from build123d import *

# Parameters (mm, degrees)
BOSS_EXTRUDE1_DEPTH = 11
SKETCH6_R           = 1
CUT_EXTRUDE7_DEPTH  = 11
SKETCH7_R           = 1
CUT_EXTRUDE8_DEPTH  = 11
SKETCH8_R           = 1
CUT_EXTRUDE9_DEPTH  = 10
CUT_EXTRUDE_START   = -6
CUT_EXTRUDE_1_DEPTH = 6
FILLET_1_R          = 2


with BuildPart() as part:
    # Sketch1 → Boss-Extrude1 (new body)
    with BuildSketch(Plane.XY):
        with BuildLine():
            Line((-54.397881045, 39.097965902), (-66.397881045, 39.097965902))
            Line((-66.397881045, 39.097965902), (-72.397881045, 33.097965902))
            Line((-72.397881045, 33.097965902), (-72.397881045, 25.597965902))
            Line((-72.397881045, 25.597965902), (-84.397881045, 25.597965902))
            ThreePointArc((-84.397881045, 25.597965902), (-85.104987826, 25.305072683), (-85.397881045, 24.597965902))
            Line((-85.397881045, 24.597965902), (-85.397881045, 18.597965902))
            ThreePointArc((-85.397881045, 18.597965902), (-85.104987826, 17.890859121), (-84.397881045, 17.597965902))
            Line((-84.397881045, 17.597965902), (-72.397881045, 17.597965902))
            Line((-72.397881045, 17.597965902), (-72.397881045, 10.097965902))
            Line((-72.397881045, 10.097965902), (-66.397881045, 4.097965902))
            Line((-66.397881045, 4.097965902), (-54.397881045, 4.097965902))
            ThreePointArc((-54.397881045, 4.097965902), (-53.690774263, 4.390859121), (-53.397881045, 5.097965902))
            Line((-53.397881045, 5.097965902), (-53.397881045, 9.097965902))
            ThreePointArc((-53.397881045, 9.097965902), (-53.690774263, 9.805072683), (-54.397881045, 10.097965902))
            Line((-54.397881045, 10.097965902), (-66.397881045, 10.097965902))
            Line((-66.397881045, 10.097965902), (-66.397881045, 33.097965902))
            Line((-66.397881045, 33.097965902), (-54.397881045, 33.097965902))
            ThreePointArc((-54.397881045, 33.097965902), (-53.690774263, 33.390859121), (-53.397881045, 34.097965902))
            Line((-53.397881045, 34.097965902), (-53.397881045, 38.097965902))
            ThreePointArc((-53.397881045, 38.097965902), (-53.690774263, 38.805072683), (-54.397881045, 39.097965902))
        make_face()
    extrude(amount=BOSS_EXTRUDE1_DEPTH)

    # Sketch6 → Cut-Extrude7 (cut)
    with BuildSketch(Plane(origin=(0, -0.303980624, 11), x_dir=(1, 0, 0), z_dir=(0, 0, 1))):
        with Locations((-59.897881045, 35.597965902)):
            Circle(SKETCH6_R)
    extrude(amount=-CUT_EXTRUDE7_DEPTH, mode=Mode.SUBTRACT)

    # Sketch7 → Cut-Extrude8 (cut)
    with BuildSketch(Plane(origin=(0, 0.204760049, 11), x_dir=(1, 0, 0), z_dir=(0, 0, 1))):
        with Locations((-59.897881045, 7.597965902)):
            Circle(SKETCH7_R)
    extrude(amount=-CUT_EXTRUDE8_DEPTH, mode=Mode.SUBTRACT)

    # Sketch8 → Cut-Extrude9 (cut)
    with BuildSketch(Plane(origin=(0, 25.597965902, 0), x_dir=(1, 0, 0), z_dir=(0, 1, 0))):
        with Locations(Location((-78.897881045, -2, 0), (0, 0, 270))):
            Circle(SKETCH8_R)
    extrude(amount=-CUT_EXTRUDE9_DEPTH, mode=Mode.SUBTRACT)

    # Эскиз1 → Вырез-Вытянуть1 (cut)
    with BuildSketch(Plane.XY.offset(11).offset(CUT_EXTRUDE_START)):
        with BuildLine():
            Line((-72.397881045, 17.597965902), (-72.397881045, 25.597965902))
            Line((-72.397881045, 25.597965902), (-84.397881045, 25.597965902))
            ThreePointArc((-84.397881045, 25.597965902), (-85.104987826, 25.305072683), (-85.397881045, 24.597965902))
            Line((-85.397881045, 24.597965902), (-85.397881045, 18.597965902))
            ThreePointArc((-85.397881045, 18.597965902), (-85.104987826, 17.890859121), (-84.397881045, 17.597965902))
            Line((-84.397881045, 17.597965902), (-72.397881045, 17.597965902))
        make_face()
    extrude(amount=CUT_EXTRUDE_1_DEPTH, mode=Mode.SUBTRACT)

    # Скругление1
    fillet_1_edges = [part.edges().sort_by_distance(p)[0] for p in [
        (-72.397881045, 10.097965902, 5.5),
        (-72.397881045, 33.097965902, 5.5),
        (-66.397881045, 39.097965902, 5.5),
        (-66.397881045, 4.097965902, 5.5),
    ]]
    fillet(fillet_1_edges, radius=FILLET_1_R)


solid = part.part
CAD build for the part. Positions are in the model's coordinates, mm. A direction names the side the tool comes from. Round coordinates to 2 decimals unless told otherwise and drop trailing zeros. Write each loop counter-clockwise with the first axis right and the second up, starting at its lowest first coordinate (ties: lowest second). Pieces come first, ordered by that corner, then holes. Notation, with made-up numbers: M 34.5,79.5 L 50.5,79.5 A17 cw 50.5,109.5 Z; hole C 56,60 d3. An arc over 180 degrees is marked long. Put each result on its own line as item: value. Start each with the question number.
1) Saw through at A-A, the plane z = 2. Count the separate pieces of the cut face and the enclosed holes in it, and give its area (3 significant figures).
2) Drill centre lines: probe 1 along Y at (x, z) = (-62, 2.5); probe 2 along X at (y, z) = (31.5, 5); probe 3 along Z at (x, y) = (-74, 22.5). Where is each one in solid material? Low to high. Write a range as [from, to].
3) Saw through at D-D, the plane y = 13. Write the cut outline in (x, z), and give its area (3 significant figures).
4) Pin check, flat tips, straight feed: pin 1 Ø5.5 at (y, z) = (19.5, 8) entering from -X; pin 2 Ø1.5 at (y, z) = (15, 3.5) entering from +X; pin 3 Ø4 at (x, y) = (-77, 21) entering from +Z; pin 4 Ø8 at (x, y) = (-81.5, 32.5) entering from +Z. Stop position of each tip, or through.
5) Saw through at B-B, the plane y = 19.5. Write the cut outline in (x, z).
6) Saw through at C-C, the plane z = 7.5. Write the cut outline in (x, y), and give its area (3 significant figures).
7) 3-axis set-ups, long thin cutter, end or side, ignore diameter. For faces 5 (the flat face through (-78, 25.598, 3)), 6 (the flat face through (-66.398, 21, 5)), 7 (the flat face through (-67, 22, 11)): which of +Z, -Z, +X, -X, +Y, -Y reach the whole face in a straight line?
8) Pull direction Y, two halves, no side cores. Call faces 1 (the flat face through (-53.398, 7, 5)), 2 (the flat face through (-69.4, 7.1, 5.4)), 3 (the cylindrical face through (-66.32, 38.95, 5.58)), 4 (the cylindrical face through (-53.7, 33.38, 5.42)): pulls with the +Y half, pulls with the -Y half, needs draft (parallel to the pull), parting line crosses it, or undercut.
Resolved:
1. separate pieces: 2
1. enclosed holes: 2
1. area: 410 mm²
2. probe 1: [4.1, 10.1], [33.1, 39.1]
2. probe 2: [-72.4, -66.4]
2. probe 3: [0, 5]
3. outline: M -72.4,0 L -66.4,0 L -66.4,11 L -72.4,11 Z
3. area: 66.0 mm²
4. pin 1: x = -72.4
4. pin 2: x = -66.4
4. pin 3: z = 5
4. pin 4: through
5. outline: M -85.4,0 L -66.4,0 L -66.4,11 L -72.4,11 L -72.4,5 L -85.4,5 Z; hole C -78.9,2 d2
6. outline: M -72.4,10.93 A2 ccw -71.81,9.51 L -66.98,4.68 A2 ccw -65.57,4.1 L -54.4,4.1 A1 ccw -53.4,5.1 L -53.4,9.1 A1 ccw -54.4,10.1 L -66.4,10.1 L -66.4,33.1 L -54.4,33.1 A1 ccw -53.4,34.1 L -53.4,38.1 A1 ccw -54.4,39.1 L -65.57,39.1 A2 ccw -66.98,38.51 L -71.81,33.68 A2 ccw -72.4,32.27 Z; hole C -59.9,7.8 d2; hole C -59.9,35.29 d2
6. area: 323 mm²
7. face 5: +Z, -Z, -X, +Y
7. face 6: +Z, -Z, +X
7. face 7: +Z, +X, -X, +Y, -Y
8. face 1: needs draft
8. face 2: pulls with the -Y half
8. face 3: pulls with the +Y half
8. face 4: undercut
